Verification items for the finished model (mm, model axes). A direction names the side the tool comes from. Give positions to 0.01 mm unless a question says otherwise; leave off trailing zeros. Loops run counter-clockwise (first coordinate to the right, second up) from the corner with the lowest first, then second, coordinate; pieces in that order, holes last. Notation, with made-up numbers: (8, -32) -> (18, -32) arc R23 cw to (18, 3) -> close; hole circle Ø8 at (17.25, 69.25). An arc over 180 degrees is marked (long way). Answer in a Markdown table with one row per item. Add a question column.
Q1. Set-up check for faces 4 (the face through (-73.35, 10.57, -44.07)), 5 (the face through (-103, 3, 2)), 6 (the face through (-104.13, 9.1, -7.83)), 7 (the face through (-1.542, 7.582, -144.874)), 8 (the face through (-75.535, 5.159, -46.502)): record each of +Z, -Z, +X, -X, +Y, -Y from which the full face is reachable in a straight line by a thin tool's end or side.
Q2. Gauge pin test, flat ends, axial feed: P1, Ø1.5, axis at x = -20, y = 4, coming from the +Z side; P2, Ø6, axis at x = -17, y = 13.5, coming from the -Z side; P3, Ø7.5, axis at x = -22, z = -125.5, coming from the +Y side; P4, Ø2, axis at x = -57.5, z = -85.5, coming from the -Y side. Record the tip position at first contact, or that the pin passes through.
Q3. Section check A-A on y = 12.5. Enter the section's corners in (x, z), and give its area (3 significant figures).
Q4. Section check D-D on z = -111.5. Enter the section's corners in (x, y), and give its area (3 significant figures).
Q5. Section check B-B on x = -72. Give the number of separate pieces and of enclosed holes in the cut face, and give its area (3 significant figures).
Q6. Release check for a two-part mould opening along X. For faces 1 (the face through (-56.568, 7.582, -96.207)), 2 (the face through (0, 9, -189.758)), 3 (the face through (-26, 3, -126)) record: pulls with the +X half, pulls with the -X half, needs draft (parallel to the pull), parting line crosses it, or undercut.
Q7. Section check C-C on x = -50.5. Enter the section's corners in (y, z).
Q8. Material ranges on probe 1 along Z at (x, y) = (-3, 6.75); probe 2 along Y at (x, z) = (-93.5, -31); probe 3 along X at (y, z) = (9, -123.5), recorded low to high.
```python
from build123d import *

# Parameters (mm, degrees)
BOSS_EXTRUDE2_DEPTH = 15.38
BOSS_EXTRUDE3_DEPTH = 1
BOSS_EXTRUDE4_DEPTH = 14.38
CUT_EXTRUDE1_DEPTH  = 8.26
SKETCH12_R          = 3.5
CUT_EXTRUDE2_DEPTH  = 8.26
CUT_EXTRUDE3_DEPTH  = 3
SKETCH16_W          = 10
SKETCH16_H          = 2
CUT_EXTRUDE4_DEPTH  = 3


with BuildPart() as part:
    # Sketch1 → Boss-Extrude2 (new body)
    with BuildSketch(Plane(origin=(0, 0, 0), x_dir=(1, 0, 0), z_dir=(0, 1, 0))):
        Polygon((-33.232050802, 130.626242439), (-11.732050802, 167.865334802), (3.267949197, 159.205080764), (-18.232050803, 121.965988402), (-18.732050803, 121.099962998), (-16.133974592, 119.599962998), (13.464101619, 170.865334801), (2.556624332, 189.757639644), (-2.556624322, 189.757639644), (-112.11324865, 2e-09), (-109.556624323, -4.428203228), (-87.74166975, -4.428203228), (-62.14359354, 39.908965344), (-64.74166975, 41.408965344), (-65.74166975, 39.676914536), (-82.74166975, 10.232050807), (-97.741669749, 18.892304845), (-80.741669749, 48.337168573), (-79.741669749, 50.069219381), (-33.732050802, 129.760217035), align=None)
        Polygon((-89.473720558, -1.42820323), (-107.824573519, -1.42820323), (-108.649147039, 0), (-99.473720558, 15.892304845), align=None, mode=Mode.SUBTRACT)
        Polygon((-9.999999996, 170.865334801), (-0.824573515, 186.757639646), (0.824573508, 186.757639646), (10.000000004, 170.865334801), align=None, mode=Mode.SUBTRACT)
    extrude(amount=BOSS_EXTRUDE2_DEPTH)

    # Sketch1_11 → Boss-Extrude3 (add)
    with BuildSketch(Plane(origin=(0, 0, 0), x_dir=(1, 0, 0), z_dir=(0, 1, 0))):
        Polygon((3.267949197, 159.205080764), (-11.732050802, 167.865334802), (-33.232050802, 130.626242439), (-18.232050803, 121.965988402), align=None)
        Polygon((-65.74166975, 39.676914536), (-80.741669749, 48.337168573), (-97.741669749, 18.892304845), (-82.74166975, 10.232050807), align=None)
    extrude(amount=BOSS_EXTRUDE3_DEPTH)

    # Sketch1_12 → Boss-Extrude4 (add)
    with BuildSketch(Plane(origin=(0, 0, 0), x_dir=(1, 0, 0), z_dir=(0, 1, 0))):
        Polygon((-33.732050802, 129.760217035), (-33.232050802, 130.626242439), (-18.232050803, 121.965988402), (-18.732050803, 121.099962998), align=None)
        Polygon((-64.74166975, 41.408965344), (-79.741669749, 50.069219381), (-80.741669749, 48.337168573), (-65.74166975, 39.676914536), align=None)
    extrude(amount=BOSS_EXTRUDE4_DEPTH)

    # Sketch10 → Cut-Extrude1 (cut)
    with BuildSketch(Plane(origin=(47.754809476, 0, -82.713756318), x_dir=(0.8660254037844418, 0, 0.49999999999999456), z_dir=(-0.4999999999999946, 0, 0.8660254037844419))):
        Polygon((-85.432921433, 3), (-81.432921433, 3), (-81.432921433, 7), (-89.432921433, 7), (-89.432921433, 3), align=None)
    extrude(amount=-CUT_EXTRUDE1_DEPTH, mode=Mode.SUBTRACT)

    # Sketch12 → Cut-Extrude2 (cut)
    with BuildSketch(Plane(origin=(1.745190528, 0, -3.022758664), x_dir=(-0.866025403784436, 0, -0.5000000000000047), z_dir=(0.5000000000000047, 0, -0.866025403784436))):
        with Locations((85.432921433, 6.5)):
            Circle(SKETCH12_R)
    extrude(amount=-CUT_EXTRUDE2_DEPTH, mode=Mode.SUBTRACT)

    # Sketch15 → Cut-Extrude3 (cut)
    with BuildSketch(Plane.XZ):
        Polygon((-87.74166975, 4.428203228), (-109.556624323, 4.428203228), (-112.11324865, -2e-09), (-101.205771363, -18.892304845), align=None)
        Polygon((13.464101619, -170.865334801), (2.556624332, -189.757639644), (-2.556624322, -189.757639644), (-13.464101609, -170.865334801), align=None)
    extrude(amount=-CUT_EXTRUDE3_DEPTH, mode=Mode.SUBTRACT)

    # Sketch16 → Cut-Extrude4 (cut)
    with BuildSketch(Plane(origin=(-84.084936489, 0, -48.546460716), x_dir=(-0.4999999999999999, 0, 0.8660254037844386), z_dir=(-0.8660254037844387, 0, -0.49999999999999994))):
        with Locations((-133.242624333, 2)):
            Rectangle(SKETCH16_W, SKETCH16_H)
        with Locations((21.128966724, 2)):
            Rectangle(SKETCH16_W, SKETCH16_H)
    extrude(amount=-CUT_EXTRUDE4_DEPTH, mode=Mode.SUBTRACT)


solid = part.part
```
Taken from the geometry:
| question | item | result |
|---|---|---|
| 1 | face 4 | +Y |
| 1 | face 5 | +Z, -X, -Y |
| 1 | face 6 | +Y, -Y |
| 1 | face 7 | +Z, +X, +Y, -Y |
| 1 | face 8 | none |
| 2 | P1 | stops at z = -121.4 |
| 2 | P2 | stops at z = -169.94 |
| 2 | P3 | stops at y = 14.38 |
| 2 | P4 | passes through |
| 3 | outline | (-112.11, 0) -> (-2.56, -189.76) -> (2.56, -189.76) -> (13.46, -170.87) -> (-16.13, -119.6) -> (-33.73, -129.76) -> (-79.74, -50.07) -> (-62.14, -39.91) -> (-87.74, 4.43) -> (-109.56, 4.43) -> close; hole (-108.65, 0) -> (-99.47, -15.89) -> (-89.47, 1.43) -> (-107.82, 1.43) -> close; hole (-97.74, -18.89) -> (-80.74, -48.34) -> (-65.74, -39.68) -> (-82.74, -10.23) -> close; hole (-33.23, -130.63) -> (-11.73, -167.87) -> (3.27, -159.21) -> (-18.23, -121.97) -> close; hole (-10, -170.87) -> (-0.82, -186.76) -> (0.82, -186.76) -> (10, -170.87) -> close |
| 3 | area | 1,460 mm² |
| 4 | outline | (-47.74, 0) -> (-44.27, 0) -> (-44.27, 15.38) -> (-47.74, 15.38) -> close |
| 4 | area | 53.3 mm² |
| 5 | separate pieces | 3 |
| 5 | enclosed holes | 0 |
| 5 | area | 217 mm² |
| 6 | face 1 | pulls with the -X half |
| 6 | face 2 | needs draft |
| 6 | face 3 | undercut |
| 7 | outline | (0, -106.72) -> (15.38, -106.72) -> (15.38, -100.72) -> (0, -100.72) -> close |
| 8 | probe 1 | z = -188.99 to -182.99, -170.87 to -162.82, -148.35 to -142.35 |
| 8 | probe 2 | y = 0 to 1, 3 to 15.38 |
| 8 | probe 3 | x = -40.81 to -37.35, -22.89 to -20.89, -17.35 to -13.88 |
